Model file for the job. Use its own axes, mm. Face numbers are marked on the shaded views. A direction names the side the tool comes from. Round coordinates to 2 decimals unless told otherwise and drop trailing zeros. Loops run counter-clockwise (first coordinate to the right, second up) from the corner with the lowest first, then second, coordinate; pieces in that order, holes last. Notation, with made-up numbers: (88.25, 61.25) -> (143.25, 61.25) arc R25 ccw to (143.25, 83.25) -> close; hole circle Ø7 at (-23, 47.25). An arc over 180 degrees is marked (long way). Use a Markdown table: item, result.
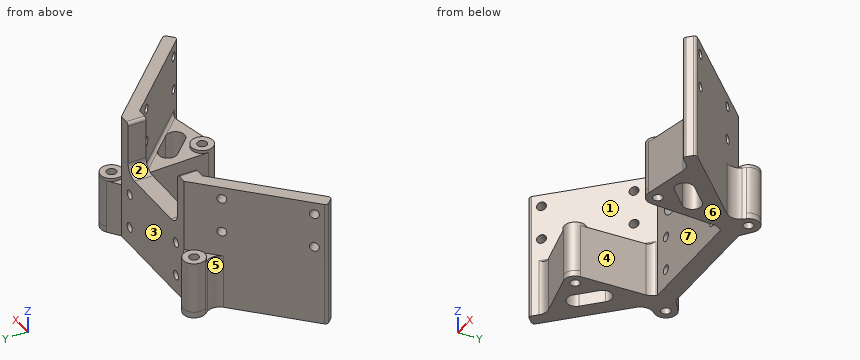
from build123d import *

# Parameters (mm, degrees)
ESQUISSE1_W             = 58
ESQUISSE1_H             = 38
ESQUISSE1_R             = 1.6
BOSS_EXTRU_1_DEPTH      = 2
BOSS_EXTRU_2_DEPTH      = 20
BOSS_EXTRU_3_DEPTH      = 20
ENL_V_MAT_EXTRU_1_DEPTH = 20
ESQUISSE6_R             = 1.5
ENL_V_MAT_EXTRU_2_DEPTH = 20
ESQUISSE7_R             = 1.5
ENL_V_MAT_EXTRU_3_DEPTH = 20
ESQUISSE8_R             = 1.5
ENL_V_MAT_EXTRU_4_DEPTH = 20
BOSS_EXTRU_5_DEPTH      = 22
ESQUISSE10_W            = 30
ESQUISSE10_H            = 18
ENL_V_MAT_EXTRU_5_DEPTH = 20
ESQUISSE11_R            = 3.6
ESQUISSE11_R_2          = 1.6
BOSS_EXTRU_6_DEPTH      = 17
BOSS_EXTRU_7_DEPTH      = 2
ESQUISSE13_R            = 1.6
BOSS_EXTRU_8_DEPTH      = 16
ENL_V_MAT_EXTRU_6_DEPTH = 16
CONG_1_R                = 4
CONG_2_R                = 1
CONG_3_R                = 1
CONG_4_R                = 1
ENL_V_MAT_EXTRU_7_DEPTH = 58.864879499


with BuildPart() as part:
    # Esquisse1 → Boss.-Extru.1 (new body)
    with BuildSketch(Plane.XY):
        Rectangle(ESQUISSE1_W, ESQUISSE1_H)
        with Locations((-25, 15)):
            Circle(ESQUISSE1_R, mode=Mode.SUBTRACT)
        with Locations((-25, -15)):
            Circle(ESQUISSE1_R, mode=Mode.SUBTRACT)
        with Locations((25, 15)):
            Circle(ESQUISSE1_R, mode=Mode.SUBTRACT)
        with Locations((25, -15)):
            Circle(ESQUISSE1_R, mode=Mode.SUBTRACT)
    extrude(amount=BOSS_EXTRU_1_DEPTH)

    # Esquisse2 → Boss.-Extru.2 (add)
    with BuildSketch(Plane.XY.offset(2)):
        Polygon((-29, -1), (-19, 9), (19, 9), (29, -1), (29, 5), (19, 15), (0, 15), (-19, 15), (-29, 5), align=None)
    extrude(amount=BOSS_EXTRU_2_DEPTH)

    # Esquisse3 → Boss.-Extru.3 (add)
    with BuildSketch(Plane.XY.offset(22)):
        Polygon((-19, 15), (-49.672555794, -15.672555794), (-46.672555794, -18.672555794), (-19, 9), (19, 9), (46.672555794, -18.672555794), (49.672555794, -15.672555794), (19, 15), align=None)
    extrude(amount=BOSS_EXTRU_3_DEPTH)

    # Esquisse4 → Enlèv. mat.-Extru.1 (cut)
    with BuildSketch(Plane.XY.offset(2)):
        with BuildLine():
            Line((-15, 9), (15, 9))
            ThreePointArc((15, 9), (19, 5), (15, 1))
            Line((15, 1), (-15, 1))
            ThreePointArc((-15, 1), (-19, 5), (-15, 9))
        make_face()
    extrude(amount=-ENL_V_MAT_EXTRU_1_DEPTH, mode=Mode.SUBTRACT)

    # Esquisse6 → Enlèv. mat.-Extru.2 (cut)
    with BuildSketch(Plane(origin=(-14, 14, 0), x_dir=(0, 0, -1), z_dir=(0.7071067811865465, -0.7071067811865487, 0))):
        with Locations(Location((-38, -42.205971521, 0), (0, 0, 90))):
            Circle(ESQUISSE6_R)
        with Locations(Location((-26.5, -14.205971521, 0), (0, 0, 90))):
            Circle(ESQUISSE6_R)
        with Locations(Location((-38, -14.205971521, 0), (0, 0, 90))):
            Circle(ESQUISSE6_R)
        with Locations(Location((-26.5, -42.205971521, 0), (0, 0, 90))):
            Circle(ESQUISSE6_R)
    extrude(amount=-ENL_V_MAT_EXTRU_2_DEPTH, mode=Mode.SUBTRACT)

    # Esquisse7 → Enlèv. mat.-Extru.3 (cut)
    with BuildSketch(Plane(origin=(14, 14, 0), x_dir=(0, 0, 1), z_dir=(-0.7071067811865464, -0.7071067811865487, 0))):
        with Locations(Location((38, -14.205971521, 0), (0, 0, 270))):
            Circle(ESQUISSE7_R)
        with Locations(Location((38, -42.205971521, 0), (0, 0, 270))):
            Circle(ESQUISSE7_R)
        with Locations(Location((26.5, -42.205971521, 0), (0, 0, 270))):
            Circle(ESQUISSE7_R)
        with Locations(Location((26.5, -14.205971521, 0), (0, 0, 270))):
            Circle(ESQUISSE7_R)
    extrude(amount=-ENL_V_MAT_EXTRU_3_DEPTH, mode=Mode.SUBTRACT)

    # Esquisse8 → Enlèv. mat.-Extru.4 (cut)
    with BuildSketch(Plane.XZ.offset(-9)):
        with Locations((-14, 17.5)):
            Circle(ESQUISSE8_R)
        with Locations((14, 17.5)):
            Circle(ESQUISSE8_R)
        with Locations((14, 6)):
            Circle(ESQUISSE8_R)
        with Locations((-14, 6)):
            Circle(ESQUISSE8_R)
    extrude(amount=-ENL_V_MAT_EXTRU_4_DEPTH, mode=Mode.SUBTRACT)

    # Esquisse9 → Boss.-Extru.5 (add)
    with BuildSketch(Plane(origin=(0, 0, 22), x_dir=(-1, 0, 0), z_dir=(0, 0, -1))):
        Polygon((49.672555794, -15.672555794), (29, 5), (29, -1), (46.672555794, -18.672555794), align=None)
        Polygon((-46.672555794, -18.672555794), (-29, -1), (-29, 5), (-49.672555794, -15.672555794), align=None)
    extrude(amount=BOSS_EXTRU_5_DEPTH)

    # Esquisse10 → Enlèv. mat.-Extru.5 (cut)
    with BuildSketch(Plane.XZ.offset(-9)):
        with Locations((0, 33)):
            Rectangle(ESQUISSE10_W, ESQUISSE10_H)
    extrude(amount=-ENL_V_MAT_EXTRU_5_DEPTH, mode=Mode.SUBTRACT)

    # Esquisse11 → Boss.-Extru.6 (add)
    with BuildSketch(Plane.XY.offset(2)):
        with Locations(Location((-25, -15, 0), (0, 0, 180))):
            Circle(ESQUISSE11_R)
        with Locations((-25, -15)):
            Circle(ESQUISSE11_R_2, mode=Mode.SUBTRACT)
        with Locations(Location((25, -15, 0), (0, 0, 180))):
            Circle(ESQUISSE11_R)
        with Locations((25, -15)):
            Circle(ESQUISSE11_R_2, mode=Mode.SUBTRACT)
        with Locations(Location((25, 15, 0), (0, 0, 180))):
            Circle(ESQUISSE11_R)
        with Locations((25, 15)):
            Circle(ESQUISSE11_R_2, mode=Mode.SUBTRACT)
        with Locations(Location((-25, 15, 0), (0, 0, 180))):
            Circle(ESQUISSE11_R)
        with Locations((-25, 15)):
            Circle(ESQUISSE11_R_2, mode=Mode.SUBTRACT)
    extrude(amount=BOSS_EXTRU_6_DEPTH)

    # Esquisse12 → Boss.-Extru.7 (add)
    with BuildSketch(Plane(origin=(0, 0, 0), x_dir=(-1, 0, 0), z_dir=(0, 0, -1))):
        Polygon((46.672555794, -18.672555794), (29, -19), (29, -1), align=None)
        Polygon((-29, -19), (-46.672555794, -18.672555794), (-29, -1), align=None)
        Polygon((29, 19), (49.672555794, -15.672555794), (29, 5), align=None)
        Polygon((-29, 19), (-29, 5), (-49.672555794, -15.672555794), align=None)
    extrude(amount=-BOSS_EXTRU_7_DEPTH)

    # Esquisse13 → Boss.-Extru.8 (add)
    with BuildSketch(Plane.XY.offset(2)):
        with BuildLine():
            ThreePointArc((-27.88, 12.84), (-27.545584412, 17.545584412), (-22.84, 17.88))
            Line((-22.84, 17.88), (-19, 15))
            Line((-19, 15), (-25, 9))
            Line((-25, 9), (-27.88, 12.84))
        make_face()
        with Locations((-25, 15)):
            Circle(ESQUISSE13_R, mode=Mode.SUBTRACT)
        with BuildLine():
            ThreePointArc((-21.4, -15), (-21.400768371, -15.07437526), (-21.403073155, -15.148718771))
            Line((-21.403073155, -15.148718771), (-20.465198865, 7.534801135))
            Line((-20.465198865, 7.534801135), (-42.785641509, -14.785641509))
            Line((-42.785641509, -14.785641509), (-25.771059191, -18.5164567))
            ThreePointArc((-25.771059191, -18.5164567), (-27.256566741, -12.195021115), (-21.4, -15))
        make_face()
        with BuildLine():
            Line((25.771059191, -18.5164567), (42.785641509, -14.785641509))
            Line((42.785641509, -14.785641509), (20.465198865, 7.534801135))
            Line((20.465198865, 7.534801135), (21.403073155, -15.148718771))
            ThreePointArc((21.403073155, -15.148718771), (24.92562474, -11.400768371), (28.6, -15))
            ThreePointArc((28.6, -15), (27.804978885, -17.256566741), (25.771059191, -18.5164567))
        make_face()
        with BuildLine():
            Line((27.88, 12.84), (25, 9))
            Line((25, 9), (19, 15))
            Line((19, 15), (22.84, 17.88))
            ThreePointArc((22.84, 17.88), (27.545584412, 17.545584412), (27.88, 12.84))
        make_face()
        with Locations((25, 15)):
            Circle(ESQUISSE13_R, mode=Mode.SUBTRACT)
    extrude(amount=BOSS_EXTRU_8_DEPTH)

    # Esquisse14 → Enlèv. mat.-Extru.6 (cut)
    with BuildSketch(Plane.XY.offset(2)):
        with BuildLine():
            Line((49.672555794, -15.672555794), (29, 19))
            Line((29, 19), (-29, 19))
            Line((-29, 19), (-49.672555794, -15.672555794))
            Line((-49.672555794, -15.672555794), (-25, 9))
            Line((-25, 9), (-27.88, 12.84))
            ThreePointArc((-27.88, 12.84), (-27.545584412, 17.545584412), (-22.84, 17.88))
            Line((-22.84, 17.88), (-19, 15))
            Line((-19, 15), (19, 15))
            Line((19, 15), (22.84, 17.88))
            ThreePointArc((22.84, 17.88), (27.545584412, 17.545584412), (27.88, 12.84))
            Line((27.88, 12.84), (25, 9))
            Line((25, 9), (49.672555794, -15.672555794))
        make_face()
        with BuildLine():
            Line((-42.785641509, -14.785641509), (-46.672555794, -18.672555794))
            Line((-46.672555794, -18.672555794), (-29, -19))
            Line((-29, -19), (29, -19))
            Line((29, -19), (46.672555794, -18.672555794))
            Line((46.672555794, -18.672555794), (42.785641509, -14.785641509))
            Line((42.785641509, -14.785641509), (25.771059191, -18.5164567))
            ThreePointArc((25.771059191, -18.5164567), (22.80186518, -17.851000405), (21.403073155, -15.148718771))
            Line((21.403073155, -15.148718771), (20.465198865, 7.534801135))
            Line((20.465198865, 7.534801135), (19, 9))
            Line((19, 9), (15, 9))
            ThreePointArc((15, 9), (19, 5), (15, 1))
            Line((15, 1), (-15, 1))
            ThreePointArc((-15, 1), (-19, 5), (-15, 9))
            Line((-15, 9), (-19, 9))
            Line((-19, 9), (-20.465198865, 7.534801135))
            Line((-20.465198865, 7.534801135), (-21.403073155, -15.148718771))
            ThreePointArc((-21.403073155, -15.148718771), (-22.80186518, -17.851000405), (-25.771059191, -18.5164567))
            Line((-25.771059191, -18.5164567), (-42.785641509, -14.785641509))
        make_face()
    extrude(amount=-ENL_V_MAT_EXTRU_6_DEPTH, mode=Mode.SUBTRACT)

    # Congé1
    cong_1_edges = [part.edges().sort_by_distance(p)[0] for p in [
        (15, 12, 24),
        (-15, 12, 24),
        (-25, 9, 9),
        (-42.785641509, -14.785641509, 9),
        (-20.465198865, 7.534801135, 9),
        (20.465198865, 7.534801135, 9),
        (42.785641509, -14.785641509, 9),
        (25, 9, 10),
    ]]
    fillet(cong_1_edges, radius=CONG_1_R)

    # Congé2
    cong_2_edges = [part.edges().sort_by_distance(p)[0] for p in [
        (-49.672555794, -15.672555794, 21),
        (-46.672555794, -18.672555794, 21),
        (46.672555794, -18.672555794, 21),
        (49.672555794, -15.672555794, 21),
    ]]
    fillet(cong_2_edges, radius=CONG_2_R)

    # Congé3
    cong_3_edges = [part.edges().sort_by_distance(p)[0] for p in [
        (15, 12, 42),
        (-15, 12, 42),
    ]]
    fillet(cong_3_edges, radius=CONG_3_R)

    # Congé4
    cong_4_edges = [part.edges().sort_by_distance(p)[0] for p in [
        (-31.847320541, -3.847320541, 18),
        (31.847320541, -3.847320541, 18),
    ]]
    fillet(cong_4_edges, radius=CONG_4_R)

    # Esquisse15 → Enlèv. mat.-Extru.7 (cut, through all)
    with BuildSketch(Plane.XY.offset(18)):
        with BuildLine():
            Line((-34.902872138, -8.3170857), (-29.246017888, -2.660231451))
            ThreePointArc((-29.246017888, -2.660231451), (-25.003377201, -2.660231451), (-25.003377201, -6.902872138))
            Line((-25.003377201, -6.902872138), (-30.660231451, -12.559726387))
            ThreePointArc((-30.660231451, -12.559726387), (-34.902872138, -12.559726387), (-34.902872138, -8.3170857))
        make_face()
        with BuildLine():
            Line((34.902872138, -8.3170857), (29.246017888, -2.660231451))
            ThreePointArc((29.246017888, -2.660231451), (25.003377201, -2.660231451), (25.003377201, -6.902872138))
            Line((25.003377201, -6.902872138), (30.660231451, -12.559726387))
            ThreePointArc((30.660231451, -12.559726387), (34.902872138, -12.559726387), (34.902872138, -8.3170857))
        make_face()
    extrude(amount=-ENL_V_MAT_EXTRU_7_DEPTH, mode=Mode.SUBTRACT)


solid = part.part
Q1. Band-saw the part on A-A, the plane z = 32.5. Give the cut face in (x, y), plus the area to 3 significant figures.
Results list:
| item | result |
|---|---|
| outline | (-48.97, -16.38) -> (-47.38, -17.97) arc R1 ccw to (-45.97, -17.97) -> (-19, 9) -> (-15, 9) -> (-15, 15) -> (-19, 15) -> (-48.97, -14.97) arc R1 ccw to start; (15, 9) -> (19, 9) -> (45.97, -17.97) arc R1 ccw to (47.38, -17.97) -> (48.97, -16.38) arc R1 ccw to (48.97, -14.97) -> (19, 15) -> (15, 15) -> close |
| area | 397 mm² |
Q2. Tool access for the marked faces 1, 2, 3 and 4: list every direction of +Z, -Z, +X, -X, +Y, -Y with a clear straight run to the whole face (end or side of a thin tool).
Results list:
| item | result |
|---|---|
| face 1 | +Z, -Y |
| face 2 | +Z, +Y, -Y |
| face 3 | +Z, -Z, +Y |
| face 4 | +Z, -Z, -Y |
Q3. Pull direction X, two halves, no side cores. Call the marked faces 5, 6 and 7: released by +X, released by -X, zero draft, split by the parting line, or undercut.
Results list:
| item | result |
|---|---|
| face 5 | released by -X |
| face 6 | zero draft |
| face 7 | undercut |
Q4. Drill centre lines: L1, parallel to Y at x = -25, z = 15; L2, parallel to Z at x = 14, y = 11.35; L3, parallel to Z at x = -34.5, y = -14.5. Where is each one in solid material? Low to high. Write a range as from..to.
Results list:
| item | result |
|---|---|
| L1 | y = -18.6..-16.6, -13.4..-6.9, -2.66..13.4, 16.6..18.6 |
| L2 | z = 0..4.5, 7.5..16, 19..25.35 |
| L3 | z = 0..18 |
Q5. Band-saw the part on B-B, the plane x = -14. Give the cut face in (y, z).
Results list:
| item | result |
|---|---|
| outline | (9, 0) -> (15, 0) -> (15, 4.5) -> (9, 4.5) -> close; (9, 7.5) -> (15, 7.5) -> (15, 16) -> (9, 16) -> close; (9, 19) -> (15, 19) -> (15, 25.35) -> (9, 25.35) -> close |
Q6. Flat gauge pins, fed straight in: pin 1 (6 mm diameter, centred on x = 26, y = 14, fed in from +Z); pin 2 (1.8 mm diameter, centred on y = 12.5, z = 36, fed in from -X); pin 3 (6.5 mm diameter, centred on x = -30, y = -9.5, fed in from +Z). Where does each tip first touch, or does it go through?
Results list:
| item | result |
|---|---|
| pin 1 | stops at z = 19 |
| pin 2 | stops at x = -22.4 |
| pin 3 | stops at z = 18 |
Q7. Band-saw the part on C-C, the plane z = 6. Give the number of separate pieces and of enclosed holes in the cut face, plus the area to 3 significant figures.
Results list:
| item | result |
|---|---|
| separate pieces | 3 |
| enclosed holes | 6 |
| area | 1,040 mm² |
